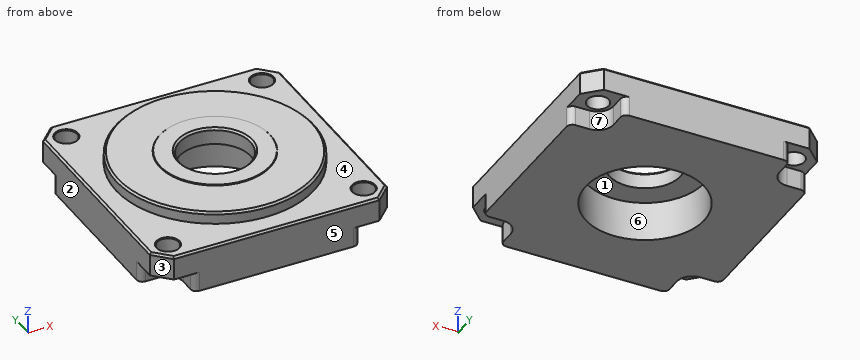
```python
from build123d import *

# Parameters (mm, degrees)
SKETCH1_W                  = 60
SKETCH1_H                  = 60
SKETCH1_R                  = 9
BOSS_EXTRUDE1_DEPTH        = 11
SKETCH2_R                  = 25
SKETCH2_R_2                = 9
BOSS_EXTRUDE2_DEPTH        = 3
SKETCH3_R                  = 14
SKETCH3_R_2                = 9
BOSS_EXTRUDE3_DEPTH        = 0.2
CHAMFER1_SIZE              = 0.5
CHAMFER2_SIZE              = 0.5
F_5_5_5_5_DIAMETER_HOLE1_D = 5.5
CIRPATTERN1_COUNT          = 4
CHAMFER3_SIZE              = 4
CHAMFER4_SIZE              = 4
CHAMFER5_SIZE              = 4
CHAMFER6_SIZE              = 4
CUT_EXTRUDE1_DEPTH         = 5
FILLET3_R                  = 1.5
FILLET4_R                  = 1.5
FILLET5_R                  = 1.5
CHAMFER7_SIZE              = 0.5
CHAMFER8_SIZE              = 0.2
CHAMFER9_SIZE              = 0.1
CHAMFER10_SIZE             = 0.5
SKETCH7_R                  = 15
CUT_EXTRUDE2_DEPTH         = 10
SCALE1_SCALE               = 2.3


with BuildPart() as part:
    # Sketch1 → Boss-Extrude1 (new body)
    with BuildSketch(Plane.XY):
        with Locations((30, 30)):
            Rectangle(SKETCH1_W, SKETCH1_H)
        with Locations((30, 30)):
            Circle(SKETCH1_R, mode=Mode.SUBTRACT)
    extrude(amount=BOSS_EXTRUDE1_DEPTH)

    # Sketch2 → Boss-Extrude2 (add)
    with BuildSketch(Plane.XY.offset(11)):
        with Locations(Location((30, 30, 0), (0, 0, 180))):
            Circle(SKETCH2_R)
        with Locations((30, 30)):
            Circle(SKETCH2_R_2, mode=Mode.SUBTRACT)
    extrude(amount=BOSS_EXTRUDE2_DEPTH)

    # Sketch3 → Boss-Extrude3 (add)
    with BuildSketch(Plane.XY.offset(14)):
        with Locations((30, 30)):
            Circle(SKETCH3_R)
        with Locations((30, 30)):
            Circle(SKETCH3_R_2, mode=Mode.SUBTRACT)
    extrude(amount=BOSS_EXTRUDE3_DEPTH)

    # Chamfer1
    chamfer1_edges = [part.edges().sort_by_distance(p)[0] for p in [
        (55, 30, 14),
    ]]
    chamfer(chamfer1_edges, length=CHAMFER1_SIZE)

    # Chamfer2
    chamfer2_edges = [part.edges().sort_by_distance(p)[0] for p in [
        (21, 30, 14.2),
    ]]
    chamfer(chamfer2_edges, length=CHAMFER2_SIZE)

    # Ø5.5 (5.5) Diameter Hole1 (through all)
    with Locations(Plane.XY.offset(11)):
        with Locations((5.251262658, 54.748737342)):
            f_5_5_5_5_diameter_hole1 = Hole(F_5_5_5_5_DIAMETER_HOLE1_D / 2)

    # CirPattern1: Ø5.5 (5.5) Diameter Hole1 ×4 about axis
    cirpattern1_axis = Axis((30, 30, 0), (0, 0, 1))
    for i in range(1, CIRPATTERN1_COUNT):
        add(f_5_5_5_5_diameter_hole1.rotate(cirpattern1_axis, i * 360 / CIRPATTERN1_COUNT), mode=Mode.SUBTRACT)

    # Chamfer3
    chamfer3_edges = [part.edges().sort_by_distance(p)[0] for p in [
        (0, 60, 5.5),
    ]]
    chamfer(chamfer3_edges, length=CHAMFER3_SIZE)

    # Chamfer4
    chamfer4_edges = [part.edges().sort_by_distance(p)[0] for p in [
        (60, 60, 5.5),
    ]]
    chamfer(chamfer4_edges, length=CHAMFER4_SIZE)

    # Chamfer5
    chamfer5_edges = [part.edges().sort_by_distance(p)[0] for p in [
        (60, 0, 5.5),
    ]]
    chamfer(chamfer5_edges, length=CHAMFER5_SIZE)

    # Chamfer6
    chamfer6_edges = [part.edges().sort_by_distance(p)[0] for p in [
        (0, 0, 5.5),
    ]]
    chamfer(chamfer6_edges, length=CHAMFER6_SIZE)

    # Sketch6 → Cut-Extrude1 (cut)
    with BuildSketch(Plane(origin=(0, 0, 0), x_dir=(-1, 0, 0), z_dir=(0, 0, -1))):
        with BuildLine():
            Line((-9, 68.337846227), (7.306259914, 68.337846227))
            Line((7.306259914, 68.337846227), (7.306259914, 51))
            Line((7.306259914, 51), (-5, 51))
            ThreePointArc((-5, 51), (-7.828427125, 52.171572875), (-9, 55))
            Line((-9, 55), (-9, 68.337846227))
        make_face()
        with BuildLine():
            Line((8.337846227, 9), (8.337846227, -7.306259914))
            Line((8.337846227, -7.306259914), (-9, -7.306259914))
            Line((-9, -7.306259914), (-9, 5))
            ThreePointArc((-9, 5), (-7.828427125, 7.828427125), (-5, 9))
            Line((-5, 9), (8.337846227, 9))
        make_face()
        with BuildLine():
            Line((-51, -8.337846227), (-67.306259914, -8.337846227))
            Line((-67.306259914, -8.337846227), (-67.306259914, 9))
            Line((-67.306259914, 9), (-55, 9))
            ThreePointArc((-55, 9), (-52.171572875, 7.828427125), (-51, 5))
            Line((-51, 5), (-51, -8.337846227))
        make_face()
        with BuildLine():
            Line((-68.337846227, 51), (-68.337846227, 67.306259914))
            Line((-68.337846227, 67.306259914), (-51, 67.306259914))
            Line((-51, 67.306259914), (-51, 55))
            ThreePointArc((-51, 55), (-52.171572875, 52.171572875), (-55, 51))
            Line((-55, 51), (-68.337846227, 51))
        make_face()
    extrude(amount=-CUT_EXTRUDE1_DEPTH, mode=Mode.SUBTRACT)

    # Fillet3
    fillet3_edges = [part.edges().sort_by_distance(p)[0] for p in [
        (60, 51, 2.5),
    ]]
    fillet(fillet3_edges, radius=FILLET3_R)

    # Fillet4
    fillet4_edges = [part.edges().sort_by_distance(p)[0] for p in [
        (51, 60, 2.5),
    ]]
    fillet(fillet4_edges, radius=FILLET4_R)

    # Fillet5
    fillet5_edges = [part.edges().sort_by_distance(p)[0] for p in [
        (9, 0, 2.5),
        (0, 9, 2.5),
        (60, 9, 2.5),
        (51, 0, 2.5),
        (9, 60, 2.5),
        (0, 51, 2.5),
    ]]
    fillet(fillet5_edges, radius=FILLET5_R)

    # Chamfer7
    chamfer7_edges = [part.edges().sort_by_distance(p)[0] for p in [
        (0, 30, 11),
        (2, 58, 11),
        (30, 60, 11),
        (58, 58, 11),
        (60, 30, 11),
        (58, 2, 11),
        (30, 0, 11),
        (2, 2, 11),
    ]]
    chamfer(chamfer7_edges, length=CHAMFER7_SIZE)

    # Chamfer8
    chamfer8_edges = [part.edges().sort_by_distance(p)[0] for p in [
        (8.001262658, 54.748737342, 11),
        (5.251262658, 8.001262658, 11),
        (51.998737342, 5.251262658, 11),
        (54.748737342, 51.998737342, 11),
    ]]
    chamfer(chamfer8_edges, length=CHAMFER8_SIZE)

    # Chamfer9
    chamfer9_edges = [part.edges().sort_by_distance(p)[0] for p in [
        (16, 30, 14.2),
    ]]
    chamfer(chamfer9_edges, length=CHAMFER9_SIZE)

    # Chamfer10
    chamfer10_edges = [part.edges().sort_by_distance(p)[0] for p in [
        (21, 30, 0),
    ]]
    chamfer(chamfer10_edges, length=CHAMFER10_SIZE)

    # Sketch7 → Cut-Extrude2 (cut)
    with BuildSketch(Plane(origin=(0, 0, 0), x_dir=(-1, 0, 0), z_dir=(0, 0, -1))):
        with Locations((-30, 30)):
            Circle(SKETCH7_R)
    extrude(amount=-CUT_EXTRUDE2_DEPTH, mode=Mode.SUBTRACT)


with BuildPart() as part_1:
    # Scale1: scaled about (30, 30, 6.673990553)
    add(part.part.scale(SCALE1_SCALE).moved(Location((-39, -39, -8.676187719))))


solid = part_1.part
```
Verification items for the finished model (mm, model axes). Face numbers are marked on the shaded views. A direction names the side the tool comes from. Give positions to 0.01 mm unless a question says otherwise; leave off trailing zeros. Write each loop counter-clockwise with the first axis right and the second up, starting at its lowest first coordinate (ties: lowest second). Pieces come first, ordered by that corner, then holes. Notation, with made-up numbers: (70, 10) - (87, 10) arc R19 cw to (87, 35) - close; hole circle Ø9 at (2, 67). An arc over 180 degrees is marked (long way). Put each result on its own line as item: value.
Q1. Section check A-A on z = 0.5. Record the cut outline in (x, y), and give its area (3 significant figures).
Result:
outline: (-39, -14.85) arc R3.45 ccw to (-35.55, -18.3) - (-27.5, -18.3) arc R9.2 cw to (-18.3, -27.5) - (-18.3, -35.55) arc R3.45 ccw to (-14.85, -39) - (74.85, -39) arc R3.45 ccw to (78.3, -35.55) - (78.3, -27.5) arc R9.2 cw to (87.5, -18.3) - (95.55, -18.3) arc R3.45 ccw to (99, -14.85) - (99, 74.85) arc R3.45 ccw to (95.55, 78.3) - (87.5, 78.3) arc R9.2 cw to (78.3, 87.5) - (78.3, 95.55) arc R3.45 ccw to (74.85, 99) - (-14.85, 99) arc R3.45 ccw to (-18.3, 95.55) - (-18.3, 87.5) arc R9.2 cw to (-27.5, 78.3) - (-35.55, 78.3) arc R3.45 ccw to (-39, 74.85) - close; hole circle Ø69 at (30, 30)
area: 13,600 mm2
Q2. Depth check by flat-ended pin: P1, Ø4, axis at x = -33.5, z = -3, coming from the -Y side; P2, Ø6.5, axis at y = 92, z = -2, coming from the +X side; P3, Ø6.5, axis at y = -32.5, z = -0.5, coming from the -X side. Enter the tip coordinate at first touch or a pass-through.
Result:
P1: y = -18.3
P2: x = 78.3
P3: x = -18.3
Q3. Section check B-B on x = 30. Record the cut outline in (y, z).
Result:
outline: (-39, -8.68) - (-4.5, -8.68) - (-4.5, 14.32) - (9.3, 14.32) - (9.3, 22.83) - (8.15, 23.98) - (-1.97, 23.98) - (-2.2, 23.75) - (-2.2, 23.52) - (-26.35, 23.52) - (-27.5, 22.37) - (-27.5, 16.62) - (-37.85, 16.62) - (-39, 15.47) - close; (50.7, 14.32) - (64.5, 14.32) - (64.5, -8.68) - (99, -8.68) - (99, 15.47) - (97.85, 16.62) - (87.5, 16.62) - (87.5, 22.37) - (86.35, 23.52) - (62.2, 23.52) - (62.2, 23.75) - (61.97, 23.98) - (51.85, 23.98) - (50.7, 22.83) - close
Q4. Section check D-D on z = 10. Record the cut outline in (x, y) (3 decimals).
Result:
outline: (-39, -29.8) - (-29.8, -39) - (89.8, -39) - (99, -29.8) - (99, 89.8) - (89.8, 99) - (-29.8, 99) - (-39, 89.8) - close; hole circle Ø12.65 at (-26.922, -26.922); hole circle Ø12.65 at (-26.922, 86.922); hole circle Ø69 at (30, 30); hole circle Ø12.65 at (86.922, -26.922); hole circle Ø12.65 at (86.922, 86.922)
Q5. Scan lines: probe 1 along Y at (x, z) = (-27, 7.5); probe 2 along Y at (x, z) = (30, 18.75); probe 3 along Y at (x, z) = (91, 9.5). Record each from-to range of solid material in increasing order. Write a range as from..to.
Result:
probe 1: -39..-33.25, -20.6..80.6, 93.25..99
probe 2: -27.5..9.3, 50.7..87.5
probe 3: -37.8..-31.76, -22.09..82.09, 91.76..97.8
Q6. Mould release check, pull along Y, two halves, no side actions. Record for the marked faces 1, 2 and 3: released by +Y, released by -Y, zero draft, split by the parting line, or undercut.
Result:
face 1: undercut
face 2: zero draft
face 3: released by -Y
Q7. Set-up check for the marked faces 4, 5, 6 and 7: record each of +Z, -Z, +X, -X, +Y, -Y from which the full face is reachable in a straight line by a thin tool's end or side.
Result:
face 4: +Z
face 5: +Z, -Z, +X, -X, -Y
face 6: -Z
face 7: -Z, +X, +Y
